CAD build for the part. Positions are in the model's coordinates, mm. Face numbers are marked on the shaded views. A direction names the side the tool comes from. Round coordinates to 2 decimals unless told otherwise and drop trailing zeros. Loops run counter-clockwise (first coordinate to the right, second up) from the corner with the lowest first, then second, coordinate; pieces in that order, holes last. Notation, with made-up numbers: M -38.5,28 L -25.5,28 A14 ccw -25.5,33 Z; hole C 65.25,87 d8. An arc over 180 degrees is marked long. Use a Markdown table: item, result. Add a question column.
(1) Band-saw the part on B-B, the plane y = 0. Write the cut outline in (x, z).
(2) Which spindle directions (+Z, -Z, +X, -X, +Y, -Y) get a long thin tool onto all of the face, cutting with end or side? Do the marked faces 1 and 2. Say none if no direction does.
(3) Band-saw the part on C-C, the plane x = 0. Write the cut outline in (y, z).
(4) Band-saw the part on A-A, the plane z = 2.5. Write the cut outline in (x, y), and give its area (3 significant figures).
(5) Flat gauge pins, fed straight in: P1, Ø1.5, axis at x = -3, z = 7, coming from the -Y side; P2, Ø5, axis at y = 7, z = 5.5, coming from the -X side; P3, Ø0.6, axis at y = 2.5, z = 5, coming from the +X side. Where does each tip first touch, or does it go through?
(6) Two-plate mould, pull along Y, no slides. Class the marked faces 3, 4 and 5: released by +Y, released by -Y, zero draft, split by the parting line, or undercut.
(7) Wall check: L1, parallel to Y at x = -0.75, z = 2.25; L2, parallel to X at y = -0.5, z = 4.5; L3, parallel to Y at x = 0.5, z = 1. Give the ranges that are in metal, low to high.
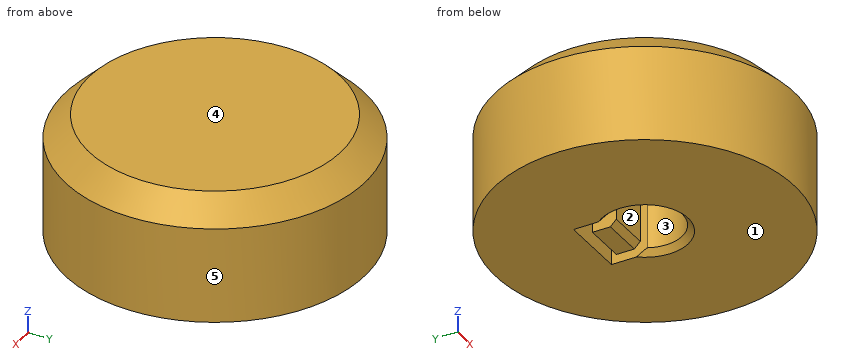
from build123d import *

# Parameters (mm, degrees)
SKETCH_R        = 12.5
PAD_DEPTH       = 10
POCKET_DEPTH    = 8
CHAMFER_SIZE    = 2
POCKET001_DEPTH = 8
CHAMFER001_SIZE = 0.5


with BuildPart() as part:
    # Sketch → Pad (new body)
    with BuildSketch(Plane.XY):
        Circle(SKETCH_R)
    extrude(amount=PAD_DEPTH)

    # Sketch001 → Pocket (cut)
    with BuildSketch(Plane.XY):
        with BuildLine():
            ThreePointArc((-2.765863, 1.4), (0, -3.1), (2.765863, 1.4))
            Line((-2.765863, 1.4), (2.765863, 1.4))
        make_face()
    extrude(amount=POCKET_DEPTH, mode=Mode.SUBTRACT)

    # Chamfer
    chamfer_edges = [part.edges().sort_by_distance(p)[0] for p in [
        (-12.5, 0, 10),
    ]]
    chamfer(chamfer_edges, length=CHAMFER_SIZE)

    # Sketch002 → Pocket001 (cut)
    with BuildSketch(Plane.XY):
        Polygon((1.75, 1.4), (1.75, 3.4), (-1.75, 3.4), (-1.75, 1.4), (-2.765863, 1.4), (-2.765863, 4.4), (2.765863, 4.4), (2.765863, 1.4), align=None)
    extrude(amount=POCKET001_DEPTH, mode=Mode.SUBTRACT)

    # Chamfer001
    chamfer001_edges = [part.edges().sort_by_distance(p)[0] for p in [
        (0, -3.1, 0),
        (0, 1.4, 0),
    ]]
    chamfer(chamfer001_edges, length=CHAMFER001_SIZE)


solid = part.part
Return value:
| question | item | result |
|---|---|---|
| 1 | outline | M -12.5,0 L -3.6,0 L -3.1,0.5 L -3.1,8 L 3.1,8 L 3.1,0.5 L 3.6,0 L 12.5,0 L 12.5,8 L 10.5,10 L -10.5,10 L -12.5,8 Z |
| 2 | face 1 | -Z, +X, -X, +Y, -Y |
| 2 | face 2 | -Z |
| 3 | outline | M -12.5,0 L -3.6,0 L -3.1,0.5 L -3.1,8 L 1.4,8 L 1.4,0.5 L 1.9,0 L 3.4,0 L 3.4,8 L 4.4,8 L 4.4,0 L 12.5,0 L 12.5,8 L 10.5,10 L -10.5,10 L -12.5,8 Z |
| 4 | outline | C 0,0 d25; M -1.75,1.4 L 1.75,1.4 L 1.75,3.4 L -1.75,3.4 Z; hole M -2.77,1.4 A3.1 ccw long 2.77,1.4 L 2.77,4.4 L -2.77,4.4 Z |
| 4 | area | 458 mm^2 |
| 5 | P1 | y = -12.3 |
| 5 | P2 | x = -11.66 |
| 5 | P3 | x = 12.3 |
| 6 | face 3 | undercut |
| 6 | face 4 | zero draft |
| 6 | face 5 | split by the parting line |
| 7 | L1 | -12.48 to -3.01, 1.4 to 3.4, 4.4 to 12.48 |
| 7 | L2 | -12.49 to -3.06, 3.06 to 12.49 |
| 7 | L3 | -12.49 to -3.06, 1.4 to 3.4, 4.4 to 12.49 |
